from build123d import *

# Parameters (mm, degrees)
BOSS_EXTRUDE4_DEPTH = 35
SKETCH11_R          = 3
CUT_EXTRUDE7_DEPTH  = 20
SKETCH12_R          = 3
CUT_EXTRUDE8_DEPTH  = 20


with BuildPart() as part:
    # Sketch9 → Boss-Extrude4 (new, symmetric)
    with BuildSketch(Plane.XY):
        with BuildLine():
            Line((19, 40), (-19, 40))
            ThreePointArc((-19, 40), (-23.242640687, 38.242640687), (-25, 34))
            Line((-25, 34), (-25, -34))
            ThreePointArc((-25, -34), (-23.242640687, -38.242640687), (-19, -40))
            Line((-19, -40), (19, -40))
            ThreePointArc((19, -40), (23.242640687, -38.242640687), (25, -34))
            Line((25, -34), (25, 34))
            ThreePointArc((25, 34), (23.242640687, 38.242640687), (19, 40))
        make_face()
        with BuildLine():
            Line((22, -34), (22, 34))
            ThreePointArc((22, 34), (21.121320344, 36.121320344), (19, 37))
            Line((19, 37), (-19, 37))
            ThreePointArc((-19, 37), (-21.121320344, 36.121320344), (-22, 34))
            Line((-22, 34), (-22, -34))
            ThreePointArc((-22, -34), (-21.121320344, -36.121320344), (-19, -37))
            Line((-19, -37), (19, -37))
            ThreePointArc((19, -37), (21.121320344, -36.121320344), (22, -34))
        make_face(mode=Mode.SUBTRACT)
    extrude(amount=BOSS_EXTRUDE4_DEPTH, both=True)

    # Sketch11 → Cut-Extrude7 (cut)
    with BuildSketch(Plane.ZY.offset(25)):
        with Locations(Location((-20, 26.5, 0), (0, 0, 270))):
            Circle(SKETCH11_R)
        with Locations(Location((20, 26.5, 0), (0, 0, 270))):
            Circle(SKETCH11_R)
        with Locations(Location((20, -26.5, 0), (0, 0, 270))):
            Circle(SKETCH11_R)
        with Locations(Location((-20, -26.5, 0), (0, 0, 270))):
            Circle(SKETCH11_R)
    extrude(amount=-CUT_EXTRUDE7_DEPTH, mode=Mode.SUBTRACT)

    # Sketch12 → Cut-Extrude8 (cut)
    with BuildSketch(Plane(origin=(25, 0, 0), x_dir=(0, 0, -1), z_dir=(1, 0, 0))):
        with Locations(Location((-9.225, 27, 0), (0, 0, 90))):
            Circle(SKETCH12_R)
        with Locations(Location((9.225, 27, 0), (0, 0, 90))):
            Circle(SKETCH12_R)
        with Locations(Location((9.225, -27, 0), (0, 0, 90))):
            Circle(SKETCH12_R)
        with Locations(Location((-9.225, -27, 0), (0, 0, 90))):
            Circle(SKETCH12_R)
    extrude(amount=-CUT_EXTRUDE8_DEPTH, mode=Mode.SUBTRACT)


solid = part.part
Read the model definition and answer for the solid it produces. Units are mm, in the model's axes. A direction names the side the tool comes from. Round coordinates to 2 decimals unless told otherwise and drop trailing zeros. Write each loop counter-clockwise with the first axis right and the second up, starting at its lowest first coordinate (ties: lowest second). Pieces come first, ordered by that corner, then holes.
1. The part is cut by section C-C, the plane x = -14. Determine the outline of the cut face in (y, z).
2. Determine the mould class of faces 1 (the face through (23.289, 38.196, 0.49)), 2 (the face through (-22, 0, 0)), 3 (the face through (-22.3, 0.2, 35)), 4 (the face through (23.196, -38.289, 0.49)) for opening direction Y: pulls with the +Y half, pulls with the -Y half, needs draft (parallel to the pull), parting line crosses it, or undercut.
3. The part is cut by section A-A, the plane z = -20. Determine the outline of the cut face in (x, y), then the cut area to 3 significant figures.
4. Given pin 1 Ø5.5 at (y, z) = (27, -9.225) entering from +X; pin 2 Ø3.5 at (y, z) = (26.5, -20) entering from -X, each flat-ended and moving along its own axis, determine where each tip first touches the part or whether it passes through.
5. Which of the six approach directions +Z, -Z, +X, -X, +Y, -Y give full straight-line access (tool end or side, diameter ignored) to faces 5 (the face through (23.521, -29.211, 11.253)), 6 (the face through (-22.3, 0.2, -35)), 7 (the face through (-23.5, -24.1, -21.8)), 8 (the face through (-21.14, -36.1, 0.49))?
6. The part is cut by section D-D, the plane z = 4. Determine the outline of the cut face in (x, y), then the cut area to 3 significant figures.
7. The part is cut by section B-B, the plane y = 31. Determine the outline of the cut face in (x, z).
8. Straight lines are drawn through the part: L1, parallel to Z at x = 22.6, y = -27 (3 decimals); L2, parallel to X at y = -21, z = -27.5; L3, parallel to Y at x = -2.5, z = 7.5. For each, find the intervals that lie inside material, in ascending order.
Values:
1. outline: (-40, -35) - (-37, -35) - (-37, 35) - (-40, 35) - close; (37, -35) - (40, -35) - (40, 35) - (37, 35) - close
2. face 1: pulls with the +Y half
2. face 2: undercut
2. face 3: needs draft
2. face 4: pulls with the -Y half
3. outline: (-25, -34) arc R6 ccw to (-19, -40) - (19, -40) arc R6 ccw to (25, -34) - (25, 34) arc R6 ccw to (19, 40) - (-19, 40) arc R6 ccw to (-25, 34) - (-25, 29.5) - (-22, 29.5) - (-22, 34) arc R3 cw to (-19, 37) - (19, 37) arc R3 cw to (22, 34) - (22, -34) arc R3 cw to (19, -37) - (-19, -37) arc R3 cw to (-22, -34) - (-22, -29.5) - (-25, -29.5) - close; (-25, -23.5) - (-22, -23.5) - (-22, 23.5) - (-25, 23.5) - close
3. area: 685 mm2
4. pin 1: stops at x = -22
4. pin 2: stops at x = 22
5. face 5: +X
5. face 6: -Z, +X, -X, +Y, -Y
5. face 7: -X
5. face 8: +Z, -Z
6. outline: (-25, -34) arc R6 ccw to (-19, -40) - (19, -40) arc R6 ccw to (25, -34) - (25, 34) arc R6 ccw to (19, 40) - (-19, 40) arc R6 ccw to (-25, 34) - close; hole (-22, -34) arc R3 ccw to (-19, -37) - (19, -37) arc R3 ccw to (22, -34) - (22, 34) arc R3 ccw to (19, 37) - (-19, 37) arc R3 ccw to (-22, 34) - close
6. area: 721 mm2
7. outline: (-25, -35) - (-22, -35) - (-22, 35) - (-25, 35) - close; (22, -35) - (25, -35) - (25, 35) - (22, 35) - close
8. L1: z = -35 to -12.225, -6.225 to 6.225, 12.225 to 35
8. L2: x = -25 to -22, 22 to 25
8. L3: y = -40 to -37, 37 to 40
